Read the model definition and answer for the solid it produces. Units are mm, in the model's axes. Face numbers are marked on the shaded views. A direction names the side the tool comes from. Round coordinates to 2 decimals unless told otherwise and drop trailing zeros. Write each loop counter-clockwise with the first axis right and the second up, starting at its lowest first coordinate (ties: lowest second). Pieces come first, ordered by that corner, then holes. Notation, with made-up numbers: (83.25, 72.25) -> (117.25, 72.25) arc R15 ccw to (117.25, 100.25) -> close; hole circle Ø10 at (14, 9). An arc over 180 degrees is marked (long way). Return JSON: item names as keys, results as strings. Group by question number.
(1) Given pin 1 (2 mm diameter, centred on x = 37.5, y = 25.5, fed in from +Z); pin 2 (6.5 mm diameter, centred on x = -51, z = 35.5, fed in from +Y); pin 3 (1.6 mm diameter, centred on x = -9, y = 0.5, fed in from +Z), each flat-ended and moving along its own axis, determine where each tip first touches the part or whether it passes through.
(2) A cutting plane is placed at C-C on z = 35.5. Give the vertices of the cut face in (x, y), then the cut area to 3 significant figures.
(3) For the marked faces 5 and 6, determine the directions among +Z, -Z, +X, -X, +Y, -Y from which every point of the face is accessible in a straight line to the end or side of a thin tool.
(4) A cutting plane is placed at B-B on x = 51. Give the vertices of the cut face in (y, z).
(5) A cutting plane is placed at D-D on y = 25. Give the vertices of the cut face in (x, z), then the cut area to 3 significant figures.
(6) Straight lines are drawn through the part: line 1 (X direction, y = 1.45, z = 35.5); line 2 (X direction, y = 9.5, z = 41.5); line 3 (Z direction, x = 51, y = 0.8). For each, find the intervals that lie inside material, in ascending order.
(7) The mould has two halves that part along X. Classify the marked faces 1, 2, 3 and 4: released by +X, released by -X, zero draft, split by the parting line, or undercut.
(8) A cutting plane is placed at A-A on z = 12. Give the vertices of the cut face in (x, y), then the cut area to 3 significant figures.
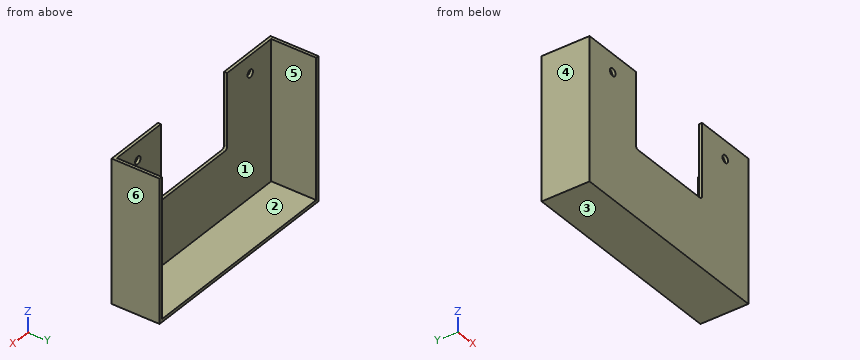
```python
from build123d import *

# Parameters (mm, degrees)
SKETCH_1_W            = 144
SKETCH_1_H            = 95
EXTRUDE_1_DEPTH       = 32
SKETCH_2_W            = 140
SKETCH_2_H            = 93
CUT_EXTRUDE_1_DEPTH   = 30
CUT_EXTRUDE_2_DEPTH   = 93.001358686
HOLE_WIZARD_5_0_5_1_D = 5


with BuildPart() as part:
    # 草图1 → 凸台-拉伸1 (new body)
    with BuildSketch(Plane.XZ):
        Rectangle(SKETCH_1_W, SKETCH_1_H)
    extrude(amount=-EXTRUDE_1_DEPTH)

    # 草图2 → 切除-拉伸1 (cut)
    with BuildSketch(Plane(origin=(0, 32, 0), x_dir=(-1, 0, 0), z_dir=(0, 1, 0))):
        with Locations((0, 1)):
            Rectangle(SKETCH_2_W, SKETCH_2_H)
    extrude(amount=-CUT_EXTRUDE_1_DEPTH, mode=Mode.SUBTRACT)

    # 草图3 → 切除-拉伸2 (cut, through all)
    with BuildSketch(Plane.XZ):
        with BuildLine():
            Line((30, 47.5), (-30, 47.5))
            Line((-30, 47.5), (-30, -0.5))
            ThreePointArc((-30, -0.5), (-29.414213562, -1.914213562), (-28, -2.5))
            Line((-28, -2.5), (28, -2.5))
            ThreePointArc((28, -2.5), (29.414213562, -1.914213562), (30, -0.5))
            Line((30, -0.5), (30, 47.5))
        make_face()
    extrude(amount=-CUT_EXTRUDE_2_DEPTH, mode=Mode.SUBTRACT)

    # Ø5.0 (5) 直径孔1 (through all)
    with Locations(Plane(origin=(0, 2, 0), x_dir=(1, 0, 0), z_dir=(0, 1, 0))):
        with Locations((51, -35.5), (-51, -35.5)):
            Hole(HOLE_WIZARD_5_0_5_1_D / 2)


solid = part.part
```
Checks:
{
 "1": {"pin 1": "stops at z = -45.5", "pin 2": "stops at y = 2", "pin 3": "stops at z = -2.5"},
 "2": {"outline": "(-72, 0) -> (-53.5, 0) -> (-53.5, 2) -> (-70, 2) -> (-70, 32) -> (-72, 32) -> close; (-48.5, 0) -> (-30, 0) -> (-30, 2) -> (-48.5, 2) -> close; (30, 0) -> (48.5, 0) -> (48.5, 2) -> (30, 2) -> close; (53.5, 0) -> (72, 0) -> (72, 32) -> (70, 32) -> (70, 2) -> (53.5, 2) -> close", "area": "268 mm^2"},
 "3": {"face 5": "+Z, +Y", "face 6": "+Z, -Z, +X, +Y, -Y"},
 "4": {"outline": "(0, -47.5) -> (32, -47.5) -> (32, -45.5) -> (2, -45.5) -> (2, 33) -> (0, 33) -> close; (0, 38) -> (2, 38) -> (2, 47.5) -> (0, 47.5) -> close"},
 "5": {"outline": "(-72, -47.5) -> (72, -47.5) -> (72, 47.5) -> (70, 47.5) -> (70, -45.5) -> (-70, -45.5) -> (-70, 47.5) -> (-72, 47.5) -> close", "area": "660 mm^2"},
 "6": {"line 1": "x = -72 to -53.5, -48.5 to -30, 30 to 48.5, 53.5 to 72", "line 2": "x = -72 to -70, 70 to 72", "line 3": "z = -47.5 to 33, 38 to 47.5"},
 "7": {"face 1": "undercut", "face 2": "undercut", "face 3": "zero draft", "face 4": "released by -X"},
 "8": {"outline": "(-72, 0) -> (-30, 0) -> (-30, 2) -> (-70, 2) -> (-70, 32) -> (-72, 32) -> close; (30, 0) -> (72, 0) -> (72, 32) -> (70, 32) -> (70, 2) -> (30, 2) -> close", "area": "288 mm^2"}
}
